from build123d import *

# Parameters (mm, degrees)
SKETCH_1_R          = 2
EXTRUDE_1_DEPTH     = 4
SKETCH_2_R          = 4
CUT_EXTRUDE_1_DEPTH = 1.3
SKETCH_3_R          = 2
CUT_EXTRUDE_2_DEPTH = 10
SKETCH_5_R          = 4
CUT_EXTRUDE_4_DEPTH = 1.3


with BuildPart() as part:
    # 草图1 → 凸台-拉伸1 (new body)
    with BuildSketch(Plane.XY):
        with BuildLine():
            Line((153.5, -28), (-153.5, -28))
            ThreePointArc((-153.5, -28), (-156.328427125, -26.828427125), (-157.5, -24))
            Line((-157.5, -24), (-157.5, 24))
            ThreePointArc((-157.5, 24), (-156.328427125, 26.828427125), (-153.5, 28))
            Line((-153.5, 28), (153.5, 28))
            ThreePointArc((153.5, 28), (156.328427125, 26.828427125), (157.5, 24))
            Line((157.5, 24), (157.5, -24))
            ThreePointArc((157.5, -24), (156.328427125, -26.828427125), (153.5, -28))
        make_face()
        with Locations((-100, 23)):
            Circle(SKETCH_1_R, mode=Mode.SUBTRACT)
        with Locations((-61.67, 23)):
            Circle(SKETCH_1_R, mode=Mode.SUBTRACT)
        with Locations((-100, -23)):
            Circle(SKETCH_1_R, mode=Mode.SUBTRACT)
        with Locations((-61.67, -23)):
            Circle(SKETCH_1_R, mode=Mode.SUBTRACT)
        with Locations((100, -23)):
            Circle(SKETCH_1_R, mode=Mode.SUBTRACT)
        with Locations((61.67, -23)):
            Circle(SKETCH_1_R, mode=Mode.SUBTRACT)
        with Locations((61.67, 23)):
            Circle(SKETCH_1_R, mode=Mode.SUBTRACT)
        with Locations((100, 23)):
            Circle(SKETCH_1_R, mode=Mode.SUBTRACT)
        with BuildLine():
            Line((-150, -12.45), (-50, -12.45))
            ThreePointArc((-50, -12.45), (-46.45, -16), (-50, -19.55))
            Line((-50, -19.55), (-150, -19.55))
            ThreePointArc((-150, -19.55), (-153.55, -16), (-150, -12.45))
        make_face(mode=Mode.SUBTRACT)
    extrude(amount=EXTRUDE_1_DEPTH)

    # 草图2 → 切除-拉伸1 (cut)
    with BuildSketch(Plane.XY.offset(4)):
        with Locations((-100, 23)):
            Circle(SKETCH_2_R)
        with Locations((-61.67, 23)):
            Circle(SKETCH_2_R)
        with Locations((-100, -23)):
            Circle(SKETCH_2_R)
        with Locations((-61.67, -23)):
            Circle(SKETCH_2_R)
        with Locations((61.67, -23)):
            Circle(SKETCH_2_R)
        with Locations((100, -23)):
            Circle(SKETCH_2_R)
        with Locations((61.67, 23)):
            Circle(SKETCH_2_R)
        with Locations((100, 23)):
            Circle(SKETCH_2_R)
    extrude(amount=-CUT_EXTRUDE_1_DEPTH, mode=Mode.SUBTRACT)

    # 草图3 → 切除-拉伸2 (cut)
    with BuildSketch(Plane.XY.offset(4)):
        with Locations((0, -16)):
            Circle(SKETCH_3_R)
    extrude(amount=-CUT_EXTRUDE_2_DEPTH, mode=Mode.SUBTRACT)

    # 草图5 → 切除-拉伸4 (cut)
    with BuildSketch(Plane(origin=(0, 0, 0), x_dir=(-1, 0, 0), z_dir=(0, 0, -1))):
        with Locations((-100, -23)):
            Circle(SKETCH_5_R)
        with Locations((-61.67, -23)):
            Circle(SKETCH_5_R)
        with Locations((61.67, -23)):
            Circle(SKETCH_5_R)
        with Locations((100, -23)):
            Circle(SKETCH_5_R)
        with Locations((100, 23)):
            Circle(SKETCH_5_R)
        with Locations((61.67, 23)):
            Circle(SKETCH_5_R)
        with Locations((-61.67, 23)):
            Circle(SKETCH_5_R)
        with Locations((-100, 23)):
            Circle(SKETCH_5_R)
    extrude(amount=-CUT_EXTRUDE_4_DEPTH, mode=Mode.SUBTRACT)


solid = part.part
Geometry check sheet. Reference: the model listing, model coordinates, mm. A direction names the side the tool comes from. Give positions to 0.01 mm unless a question says otherwise; leave off trailing zeros. Order: outer loops, then holes, each group sorted by start corner. A loop starts at its lowest first (then second) coordinate and runs counter-clockwise, first axis right, second up.
1) Material ranges on probe 1 along X at (y, z) = (23.5, 2.6); probe 2 along Y at (x, z) = (-100, 0.75); probe 3 along Y at (x, z) = (-143, 2.05), recorded low to high.
Results are:
probe 1: x = -157.5 to -101.94, -98.06 to -63.61, -59.73 to 59.73, 63.61 to 98.06, 101.94 to 157.5
probe 2: y = -28 to -27, -12.45 to 19, 27 to 28
probe 3: y = -28 to -19.55, -12.45 to 28
2) Tool access check on faces 3 (the cylindrical face through (103.815, 24.201, 3.359)), 4 (the cylindrical face through (-61.524, -26.997, 0.641)). Record the directions out of +Z, -Z, +X, -X, +Y, -Y that give a thin tool (end or side, any length) a straight path to the whole face; none if there is none.
Results are:
face 3: +Z
face 4: -Z
3) Cross-section at A-A (x = -53.5). Record the boundary of the cut face in (y, z).
Results are:
outline: (-28, 0) - (-19.55, 0) - (-19.55, 4) - (-28, 4) - close; (-12.45, 0) - (28, 0) - (28, 4) - (-12.45, 4) - close
4) Draft check along X on faces 1 (the cylindrical face through (-61.816, -26.997, 3.359)), 2 (the flat face through (2, 0, 4)). Enter one of: released by +X, released by -X, zero draft, split by the parting line, or undercut.
Results are:
face 1: undercut
face 2: zero draft
5) Gauge pin test, flat ends, axial feed: pin 1 (6.5 mm diameter, centred on x = 61.67, y = 23, fed in from -Z); pin 2 (2.5 mm diameter, centred on x = 100, y = 23, fed in from -Z) (3 decimals); pin 3 (5 mm diameter, centred on x = 100, y = 23, fed in from +Z). Record the tip position at first contact, or that the pin passes through.
Results are:
pin 1: stops at z = 1.3
pin 2: passes through
pin 3: stops at z = 2.7
